```python
from build123d import *

# Parameters (mm, degrees)
SKETCH1_R                      = 14.681199999999999
SKETCH1_R_2                    = 11.5062
BEARING_INSERT_EXTRUDE_DEPTH   = 4.7625
APEX_SLOT_INSERT_EXTRUDE_DEPTH = 3.175
FILLET1_R                      = 16.002
FILLET2_R                      = 1.5875


with BuildPart() as part:
    # Sketch1 → Bearing_Insert_Extrude (new, symmetric)
    with BuildSketch(Plane(origin=(0, 0, 0), x_dir=(1, 0, 0), z_dir=(0, 1, 0))):
        with Locations(Location((0, 0, 0), (0, 0, 90))):
            Circle(SKETCH1_R)
        with Locations(Location((0, 0, 0), (0, 0, 90))):
            Circle(SKETCH1_R_2, mode=Mode.SUBTRACT)
    extrude(amount=BEARING_INSERT_EXTRUDE_DEPTH, both=True)

    # Sketch1<4> → Apex_Slot_Insert_Extrude (add, symmetric)
    with BuildSketch(Plane(origin=(0, 0, 0), x_dir=(1, 0, 0), z_dir=(0, 1, 0))):
        with BuildLine():
            Line((-10.318749999999993, -10.443228996699254), (-10.318749999999994, -49.390299999999996))
            Line((-10.318749999999994, -49.390299999999996), (10.318750000000005, -49.39029999999999))
            Line((10.318750000000005, -49.39029999999999), (10.318750000000005, -26.704691888242454))
            Line((10.318750000000003, -26.704691888242454), (25.572760300589366, -43.49611782976841))
            Line((25.572760300589366, -43.49611782976841), (40.84821825442049, -29.619274148630485))
            Line((40.84821825442049, -29.619274148630485), (14.659851632931186, -0.7914439591308806))
            ThreePointArc((14.659851632931188, -0.7914439591308853), (5.291552650188477, -13.694418716772292), (-10.318749999999994, -10.443228996699252))
        make_face()
        with BuildLine():
            ThreePointArc((5.556250000000003, -39.07155000000002), (3.51e-15, -44.62780000000001), (-5.556249999999994, -39.07155000000002))
            Line((-5.556249999999995, -39.07155000000002), (-5.556249999999993, -25.482550000000018))
            ThreePointArc((-5.556249999999995, -25.482550000000018), (4.34e-15, -19.92630000000002), (5.556250000000002, -25.482550000000018))
            Line((5.556250000000002, -25.482550000000018), (5.556250000000004, -39.07155000000002))
        make_face(mode=Mode.SUBTRACT)
        with BuildLine():
            ThreePointArc((30.384690732198205, -25.183893713515992), (30.00814073570387, -33.0325903075461), (22.159444141673756, -32.65604031105178))
            Line((22.159444141673756, -32.65604031105178), (13.022076302401407, -22.59773876606759))
            ThreePointArc((13.022076302401405, -22.59773876606759), (13.398626298895733, -14.749042172037479), (21.247322892925844, -15.125592168531803))
            Line((21.247322892925844, -15.125592168531803), (30.384690732198205, -25.18389371351599))
        make_face(mode=Mode.SUBTRACT)
    extrude(amount=APEX_SLOT_INSERT_EXTRUDE_DEPTH, both=True)

    # Fillet1
    fillet1_edges = [part.edges().sort_by_distance(p)[0] for p in [
        (14.659851632931186, 0, 0.791443959130883),
        (-10.318749999999994, 0, 10.443228996699252),
    ]]
    fillet(fillet1_edges, radius=FILLET1_R)

    # Fillet2
    fillet2_edges = [part.edges().sort_by_distance(p)[0] for p in [
        (-10.318749999999994, 0, 49.390299999999996),
        (10.318750000000005, 0, 49.39029999999999),
        (10.318750000000005, 0, 26.704691888242454),
        (25.572760300589366, 0, 43.49611782976841),
        (40.84821825442049, 0, 29.619274148630485),
    ]]
    fillet(fillet2_edges, radius=FILLET2_R)


solid = part.part
```
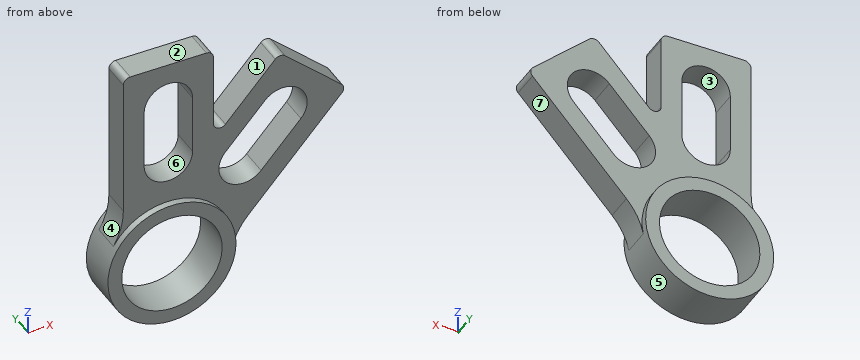
Geometry check sheet. Reference: the model listing, model coordinates, mm. Face numbers are marked on the shaded views. A direction names the side the tool comes from. Coordinates: 2 decimals unless noted, no trailing zeros. Loops run counter-clockwise (first coordinate to the right, second up) from the corner with the lowest first, then second, coordinate; pieces in that order, holes last. Notation, with made-up numbers: (87, 26) - (116, 26) arc R28 ccw to (116, 50) - close; hole circle Ø5 at (75, 21). An arc over 180 degrees is marked (long way). One line per item, written item: value. Start each with the question number.
(1) Depth check by flat-ended pin: P1, Ø3, axis at y = 1.5, z = 38, coming from the +X side; P2, Ø3, axis at y = 1, z = 34, coming from the -X side; P3, Ø5, axis at x = 7, z = 21.5, coming from the -Y side (3 decimals). Enter the tip coordinate at first touch or a pass-through.
(2) Cross-section at C-C on x = 28. Enter the section's corners in (y, z) (3 decimals), plus the area to 3 significant figures.
(3) Cross-section at A-A on y = 1. Enter the section's corners in (x, z) (1 decimal).
(4) Cross-section at D-D on z = 0. Enter the section's corners in (x, y) (1 decimal).
(5) Mould release check, pull along Z, two halves, no side actions. Record for the marked faces 4, 5, 6 and 7: released by +Z, released by -Z, zero draft, split by the parting line, or undercut.
(6) Material ranges on line 1 (X direction, y = 1, z = 24); line 2 (Z direction, x = -1, y = 1); line 3 (Y direction, x = -7, z = 42.5) (3 decimals), recorded low to high. Write a range as [from, to].
(7) Tool access check on the marked faces 1, 2 and 3. Record the directions out of +Z, -Z, +X, -X, +Y, -Y that give a thin tool (end or side, any length) a straight path to the whole face; none if there is none.
(8) Cross-section at B-B on x = 0. Enter the section's corners in (y, z) (1 decimal).
Results below:
1. P1: stops at x = 33.27
1. P2: stops at x = -10.32
1. P3: stops at y = -3.175
2. outline: (-3.175, 15.476) - (3.175, 15.476) - (3.175, 22.559) - (-3.175, 22.559) - close; (-3.175, 34.201) - (3.175, 34.201) - (3.175, 41.291) - (-3.175, 41.291) - close
2. area: 90.0 mm2
3. outline: (-12.6, 7.5) arc R14.7 ccw (long way) to (14.4, -2.9) arc R16 cw to (18.2, 4.7) - (39.8, 28.4) arc R1.6 ccw to (39.7, 30.7) - (26.7, 42.4) arc R1.6 ccw to (24.5, 42.3) - (13.1, 29.7) arc R1.6 cw to (10.3, 30.8) - (10.3, 47.8) arc R1.6 ccw to (8.7, 49.4) - (-8.7, 49.4) arc R1.6 ccw to (-10.3, 47.8) - (-10.3, 15.8) arc R16 cw to start; hole circle Ø23 at (0, 0); hole (-5.6, 25.5) arc R5.6 ccw to (5.6, 25.5) - (5.6, 39.1) arc R5.6 ccw to (-5.6, 39.1) - close; hole (13, 22.6) arc R5.6 ccw to (21.2, 15.1) - (30.4, 25.2) arc R5.6 ccw to (22.2, 32.7) - close
4. outline: (-14.7, -4.8) - (-11.5, -4.8) - (-11.5, 4.8) - (-14.7, 4.8) - close; (11.5, -4.8) - (14.7, -4.8) - (14.7, -3.2) - (15.3, -3.2) - (15.3, 3.2) - (14.7, 3.2) - (14.7, 4.8) - (11.5, 4.8) - close
5. face 4: released by +Z
5. face 5: split by the parting line
5. face 6: undercut
5. face 7: released by -Z
6. line 1: x = [-10.32, -5.35], [5.35, 14.3], [29.31, 35.74]
6. line 2: z = [-14.65, -11.46], [11.46, 20.02], [44.54, 49.39]
6. line 3: y = [-3.175, 3.175]
7. face 1: +Z, +Y, -Y
7. face 2: +Z, +X, -X, +Y, -Y
7. face 3: +Y, -Y
8. outline: (-4.8, -14.7) - (4.8, -14.7) - (4.8, -11.5) - (-4.8, -11.5) - close; (-4.8, 11.5) - (4.8, 11.5) - (4.8, 14.7) - (3.2, 14.7) - (3.2, 19.9) - (-3.2, 19.9) - (-3.2, 14.7) - (-4.8, 14.7) - close; (-3.2, 44.6) - (3.2, 44.6) - (3.2, 49.4) - (-3.2, 49.4) - close
